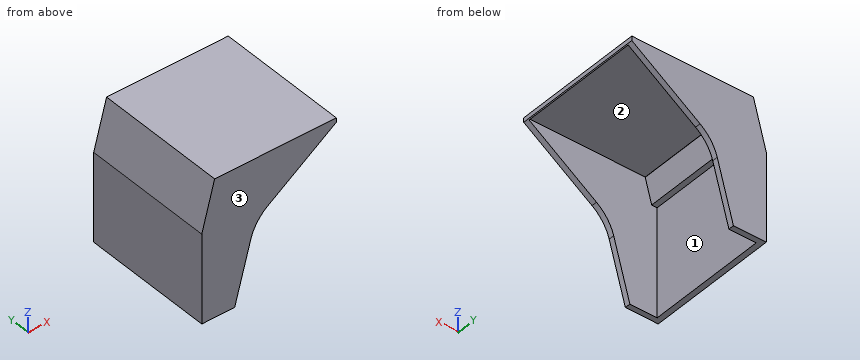
```python
from build123d import *

# Parameters (mm, degrees)
F1_DEPTH  = 120
F2_W      = 85.2778990954
F2_H      = 80
F3_DEPTH  = 98
F6_DEPTH  = 80
F7_W      = 105
F7_H      = 80
F8_DEPTH  = 120
F9_DEPTH  = 15
F10_DEPTH = 30
F11_DEPTH = 15


with BuildPart() as f1:
    # F0 (on Front) → F1 (new body)
    with BuildSketch(Plane.XZ):
        with BuildLine():
            Line((0, 80), (0, 0))
            Line((0, 0), (29.7221009046, 0))
            Line((29.7221009046, 0), (44.3633417849, 53.6774845415))
            ThreePointArc((44.3633417849, 53.6774845415), (50.1903143406, 66.0986305535), (59.871849565, 75.8200683645))
            Line((59.871849565, 75.8200683645), (121.6468570296, 119.466662183))
            Line((121.6468570296, 119.466662183), (121.6468570296, 123.466662183))
            Line((121.6468570296, 123.466662183), (11.6468570296, 123.466662183))
            Line((11.6468570296, 123.466662183), (0, 80))
        make_face()
    extrude(amount=F1_DEPTH)

    # F2 (on face) → F3 (cut)
    with BuildSketch(Plane(origin=(0, 0, 0), x_dir=(1, 0, 0), z_dir=(0, 0, -1))):
        with Locations((72.3610504523, 60)):
            Rectangle(F2_W, F2_H)
        Polygon((5, 100), (5, 60), (5, 20), (29.7221009046, 20), (29.7221009046, 100), align=None)
    extrude(amount=-F3_DEPTH, mode=Mode.SUBTRACT)

    # F5 (on offset) → F6 (cut)
    with BuildSketch(Plane(origin=(-15.1703708686, 0, 4.0648886231), x_dir=(0, -1, 0), z_dir=(-0.9659258263, 0, 0.2588190451))):
        Polygon((115, 79.7740661031), (115, 99.7740661031), (115, 119.7740661031), (35, 119.7740661031), (35, 79.7740661031), align=None)
    extrude(amount=-F6_DEPTH, mode=Mode.SUBTRACT)

    # F7 (on Top) → F8 (cut)
    with BuildSketch(Plane.XY):
        with Locations((68.3294385483, -75)):
            Rectangle(F7_W, F7_H)
    extrude(amount=F8_DEPTH, mode=Mode.SUBTRACT)

    # F9 (cut): a face of the model
    f9_faces = [f1.faces().sort_by_distance(p)[0] for p in [
        (29.9652985241, -20, 58.8911596381),
    ]]
    extrude(f9_faces, amount=-F9_DEPTH, mode=Mode.SUBTRACT)

    # F10 (cut): a face of the model
    f10_faces = [f1.faces().sort_by_distance(p)[0] for p in [
        (60.278784087, -35, 109.488672273),
    ]]
    extrude(f10_faces, amount=-F10_DEPTH, mode=Mode.SUBTRACT)

    # F11 (cut): a face of the model
    f11_faces = [f1.faces().sort_by_distance(p)[0] for p in [
        (10.1941550896, -100, 42.5407610302),
    ]]
    extrude(f11_faces, amount=-F11_DEPTH, mode=Mode.SUBTRACT)


solid = f1.part
```
Verification items for the finished model (mm, model axes). Face numbers are marked on the shaded views. Coordinates: 2 decimals unless noted, no trailing zeros. Order: outer loops, then holes, each group sorted by start corner. A loop starts at its lowest first (then second) coordinate and runs counter-clockwise, first axis right, second up. Notation, with made-up numbers: (45.5, 47.25) -> (59.5, 47.25) arc R25 ccw to (59.5, 83.25) -> close; hole circle Ø3 at (70.25, 62.5). An arc over 180 degrees is marked (long way). Put each result on its own line as item: value. Start each with the question number.
1) Release check for a two-part mould opening along X. For the marked faces 1, 2 and 3 record: pulls with the +X half, pulls with the -X half, needs draft (parallel to the pull), parting line crosses it, or undercut.
2) Material ranges on L1, parallel to Y at x = 37, z = 69.5; L2, parallel to X at y = -110.5, z = 18.5; L3, parallel to Z at x = 35.5, y = -105, recorded low to high.
3) Cross-section at A-A (x = 24). Enter the section's corners in (y, z), plus the area to 3 significant figures.
4) Go/stop test with flat-tipped pins: pin 1 (8 mm diameter, centred on y = -96.5, z = 36, fed in from -X); pin 2 (5 mm diameter, centred on y = -98.5, z = 77, fed in from +X); pin 3 (5 mm diameter, centred on x = 49, y = -102, fed in from -Z); pin 4 (1.5 mm diameter, centred on x = 7, y = -55, fed in from -Z). Record where each tip stops, or that it passes through.
5) Cross-section at C-C (z = 42). Enter the section's corners in (x, y).
6) Cross-section at B-B (y = -111.5). Enter the section's corners in (x, z), plus the area to 3 significant figures.
Geometry check:
1. face 1: pulls with the +X half
1. face 2: undercut
1. face 3: needs draft
2. L1: y = -120 to -115, -5 to 0
2. L2: x = 0 to 5
2. L3: z = 120 to 123.47
3. outline: (-120, 0) -> (-115, 0) -> (-115, 120) -> (-5, 120) -> (-5, 0) -> (0, 0) -> (0, 123.47) -> (-120, 123.47) -> close
3. area: 1,620 mm^2
4. pin 1: stops at x = 0
4. pin 2: stops at x = 5
4. pin 3: stops at z = 120
4. pin 4: stops at z = 98
5. outline: (0, -120) -> (41.18, -120) -> (41.18, -115) -> (5, -115) -> (5, -5) -> (41.18, -5) -> (41.18, 0) -> (0, 0) -> close
6. outline: (0, 0) -> (5, 0) -> (5, 98) -> (10, 98) -> (15.83, 119.76) -> (15.83, 120) -> (120.83, 120) -> (120.83, 118.89) -> (121.65, 119.47) -> (121.65, 123.47) -> (11.65, 123.47) -> (0, 80) -> close
6. area: 944 mm^2
